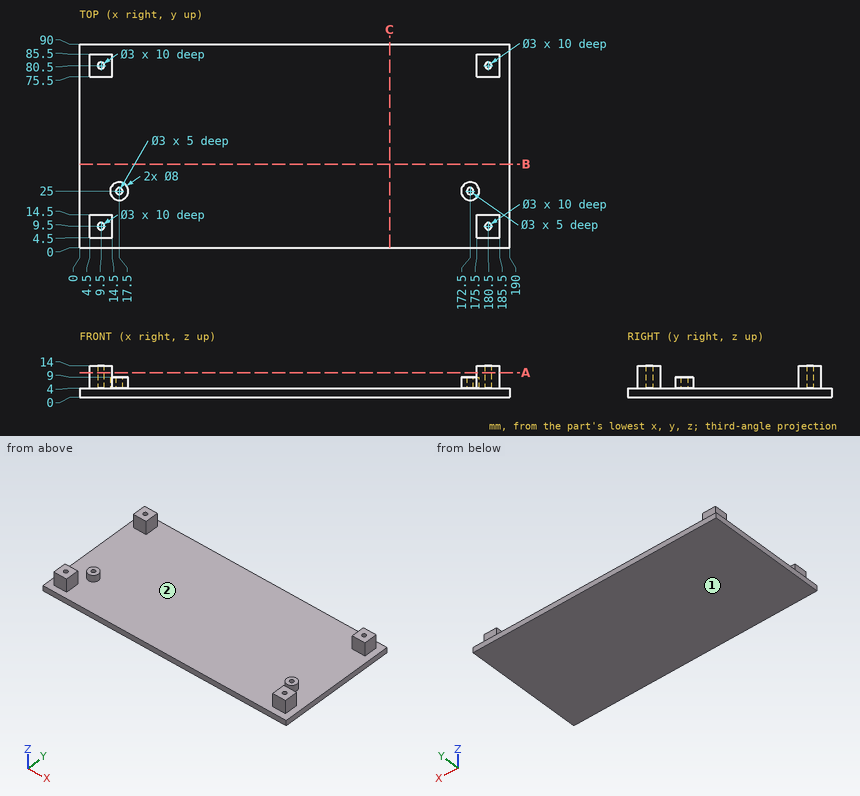
Check sheet for the drawn part. Datum: minimum x, y, z corner. Units: mm. Round coordinates to 2 decimals unless told otherwise and drop trailing zeros. Loops run counter-clockwise (first coordinate to the right, second up) from the corner with the lowest first, then second, coordinate; pieces in that order, holes last. Notation, with made-up numbers: (10.25, -10) - (27.25, -10) arc R19 cw to (27.25, 20) - close; hole circle Ø4 at (48.5, 20.25). An arc over 180 degrees is marked (long way). Write each question's results on one line, items separated by ' | '. Start each with the question number.
Q1. Release check for a two-part mould opening along X. For the marked faces 1 and 2 record: +X half, -X half, draft (parallel to the pull), parting line (faces both ways), or undercut.
Q2. Cross-section at A-A on z = 11. Enter the section's corners in (x, y).
Q3. Thickness scan on line 1 (Y direction, x = 9.5, z = 10.25); line 2 (X direction, y = 80.5, z = 8.25); line 3 (X direction, y = 10, z = 8.75). Record the ranges inside material, lowest first. Write a range as [from, to].
Q4. Gauge pin test, flat ends, axial feed: P1, Ø3, axis at x = 55, y = 15.5, coming from the +Z side; P2, Ø5, axis at x = 11, z = 7.5, coming from the -Y side; P3, Ø3.5, axis at x = 172, y = 25.5, coming from the +Z side; P4, Ø1, axis at x = 154, z = 5, coming from the +Y side. Record the tip position at first contact, or that the pin passes through.
Q5. Cross-section at C-C on x = 137. Enter the section's corners in (y, z), and give its area (3 significant figures).
Q6. Cross-section at B-B on y = 37. Enter the section's corners in (x, z), and give its area (3 significant figures).
Answers below:
1) face 1: draft | face 2: undercut
2) outline: (4.5, 4.5) - (14.5, 4.5) - (14.5, 14.5) - (4.5, 14.5) - close; (4.5, 75.5) - (14.5, 75.5) - (14.5, 85.5) - (4.5, 85.5) - close; (175.5, 4.5) - (185.5, 4.5) - (185.5, 14.5) - (175.5, 14.5) - close; (175.5, 75.5) - (185.5, 75.5) - (185.5, 85.5) - (175.5, 85.5) - close; hole circle Ø3 at (9.5, 9.5); hole circle Ø3 at (9.5, 80.5); hole circle Ø3 at (180.5, 9.5); hole circle Ø3 at (180.5, 80.5)
3) line 1: y = [4.5, 8], [11, 14.5], [75.5, 79], [82, 85.5] | line 2: x = [4.5, 8], [11, 14.5], [175.5, 179], [182, 185.5] | line 3: x = [4.5, 8.09], [10.91, 14.5], [175.5, 179.09], [181.91, 185.5]
4) P1: stops at z = 4 | P2: stops at y = 4.5 | P3: stops at z = 9 | P4: passes through
5) outline: (0, 0) - (90, 0) - (90, 4) - (0, 4) - close | area: 360 mm²
6) outline: (0, 0) - (190, 0) - (190, 4) - (0, 4) - close | area: 760 mm²
